```python
from build123d import *

# Parameters (mm, degrees)
SKETCH1_R           = 32.5
SKETCH1_R_2         = 22.5
BOSS_EXTRUDE1_DEPTH = 35
SKETCH2_W           = 7
SKETCH2_H           = 14
CUT_EXTRUDE1_DEPTH  = 84.740671122
CIRPATTERN1_COUNT   = 2
CIRPATTERN1_ANGLE   = 90


with BuildPart() as part:
    # Sketch1 → Boss-Extrude1 (new, symmetric)
    with BuildSketch(Plane(origin=(0, 0, 0), x_dir=(1, 0, 0), z_dir=(0, 1, 0))):
        with Locations(Location((0, 0, 0), (0, 0, 270))):
            Circle(SKETCH1_R)
        with Locations(Location((0, 0, 0), (0, 0, 270))):
            Circle(SKETCH1_R_2, mode=Mode.SUBTRACT)
    extrude(amount=BOSS_EXTRUDE1_DEPTH, both=True)

    # Sketch2 → Cut-Extrude1 (cut, through all)
    with BuildSketch(Plane(origin=(0, 35, 0), x_dir=(1, 0, 0), z_dir=(0, 1, 0))):
        with Locations((21.6, 0)):
            Rectangle(SKETCH2_W, SKETCH2_H)
    cut_extrude1 = extrude(amount=-CUT_EXTRUDE1_DEPTH, mode=Mode.SUBTRACT)

    # CirPattern1: Cut-Extrude1 ×2 about axis
    cirpattern1_axis = Axis((0, 0, 0), (0, 1, 0))
    for i in range(1, CIRPATTERN1_COUNT):
        add(cut_extrude1.rotate(cirpattern1_axis, i * CIRPATTERN1_ANGLE / (CIRPATTERN1_COUNT - 1)), mode=Mode.SUBTRACT)


solid = part.part
```
Source: CAD feature listing. Evaluate the final solid. Frame: model axes, mm. A direction names the side the tool comes from. Give positions to 0.01 mm unless a question says otherwise; leave off trailing zeros. Write each loop counter-clockwise with the first axis right and the second up, starting at its lowest first coordinate (ties: lowest second). Pieces come first, ordered by that corner, then holes. Notation, with made-up numbers: (15.5, 84.25) - (40.5, 84.25) arc R18 cw to (40.5, 96.25) - close; hole circle Ø5 at (-7.75, 55). An arc over 180 degrees is marked (long way). One line per item, written item: value. Start each with the question number.
Q1. Section query A-A, the plane x = 0. Return the cut outline in (y, z), then the cut area to 3 significant figures.
Q2. Material intervals for probe 1 along X at (y, z) = (13, 0); probe 2 along Z at (x, y) = (0.5, -5.5); probe 3 along X at (y, z) = (-21, 11), sorted ascending. Write a range as from..to.
Q3. Section query C-C, the plane y = 20. Return the cut outline in (x, z), then the cut area to 3 significant figures.
Q4. Set-up query: faces 1 (the face through (-14, 35, 21)), 2 (the face through (25.1, 0, 0)). Return all of +Z, -Z, +X, -X, +Y, -Y with unobstructed straight access to the full face (end or side cutting, diameter ignored); none if empty.
Q5. First-contact query: pin 1 Ø11 at (y, z) = (-11, 1.5) entering from -X; pin 2 Ø12 at (x, y) = (-9, -27.5) entering from -Z; pin 3 Ø5 at (x, y) = (-9, 22.5) entering from +Z. Flat tips, straight axial feed; report the tip coordinate or a pass-through.
Q6. Section query D-D, the plane x = -26.5. Return the cut outline in (y, z).
Q7. Draft query along Z for faces 3 (the face through (0, 0, -25.1)), 4 (the face through (-14, -35, 21)), 5 (the face through (9.76, 0.49, 31)). Return one class per face: +Z half, -Z half, draft (parallel to the pull), parting line (faces both ways), or undercut.
Q8. Section query B-B, the plane z = 0. Return the cut outline in (x, y), then the cut area to 3 significant figures.
Answer:
1. outline: (-35, -32.5) - (35, -32.5) - (35, -25.1) - (-35, -25.1) - close; (-35, 22.5) - (35, 22.5) - (35, 32.5) - (-35, 32.5) - close
1. area: 1,220 mm2
2. probe 1: x = -32.5..-22.5, 25.1..32.5
2. probe 2: z = -32.5..-25.1, 22.49..32.5
2. probe 3: x = -30.58..-19.63, 19.63..30.58
3. outline: circle Ø65 at (0, 0); hole (-7, -25.1) - (7, -25.1) - (7, -21.38) arc R22.5 ccw to (21.38, -7) - (25.1, -7) - (25.1, 7) - (21.38, 7) arc R22.5 ccw (long way) to (-7, -21.38) - close
3. area: 1,640 mm2
4. face 1: +Z, -Z, +X, -X, +Y
4. face 2: +Y, -Y
5. pin 1: stops at x = -32.5
5. pin 2: stops at z = -32.36
5. pin 3: stops at z = 31.84
6. outline: (-35, -18.81) - (35, -18.81) - (35, 18.81) - (-35, 18.81) - close
7. face 3: undercut
7. face 4: draft
7. face 5: parting line
8. outline: (-32.5, -35) - (-22.5, -35) - (-22.5, 35) - (-32.5, 35) - close; (25.1, -35) - (32.5, -35) - (32.5, 35) - (25.1, 35) - close
8. area: 1,220 mm2
